Could you check a few things on this model? Use its own coordinates, in mm. Coordinates: 2 decimals unless noted, no trailing zeros. Loops run counter-clockwise (first coordinate to the right, second up) from the corner with the lowest first, then second, coordinate; pieces in that order, holes last. Notation, with made-up numbers: (82.25, 48.25) - (108.25, 48.25) arc R9 cw to (108.25, 62.25) - close; hole circle Ø5 at (54, 69). An arc over 180 degrees is marked (long way). Put each result on its own line as item: value. Start each with the question number.
```python
from build123d import *

# Parameters (mm, degrees)
SKETCH1_W           = 90
SKETCH1_H           = 60
SKETCH1_R           = 4.8
SKETCH1_R_2         = 2.55
BOSS_EXTRUDE1_DEPTH = 6.35
SKETCH3_R           = 1.25
CUT_EXTRUDE1_DEPTH  = 8


with BuildPart() as part:
    # Sketch1 → Boss-Extrude1 (new body)
    with BuildSketch(Plane(origin=(0, 0, 0), x_dir=(1, 0, 0), z_dir=(0, 1, 0))):
        Rectangle(SKETCH1_W, SKETCH1_H)
        with Locations((-37.5, 0)):
            Circle(SKETCH1_R, mode=Mode.SUBTRACT)
        with Locations((37.5, 0)):
            Circle(SKETCH1_R, mode=Mode.SUBTRACT)
        with Locations((-23.6, -23.6)):
            Circle(SKETCH1_R_2, mode=Mode.SUBTRACT)
        with Locations((23.6, -23.6)):
            Circle(SKETCH1_R_2, mode=Mode.SUBTRACT)
        with Locations((23.6, 23.6)):
            Circle(SKETCH1_R_2, mode=Mode.SUBTRACT)
        with Locations((-23.6, 23.6)):
            Circle(SKETCH1_R_2, mode=Mode.SUBTRACT)
    extrude(amount=BOSS_EXTRUDE1_DEPTH)

    # Sketch3 → Cut-Extrude1 (cut)
    with BuildSketch(Plane(origin=(0, 6.35, 0), x_dir=(1, 0, 0), z_dir=(0, 1, 0))):
        with Locations((-11, 0)):
            Circle(SKETCH3_R)
        with Locations((11, 0)):
            Circle(SKETCH3_R)
    extrude(amount=-CUT_EXTRUDE1_DEPTH, mode=Mode.SUBTRACT)


solid = part.part
```
(1) If we mould it in two halves opening along Z, with no side actions, what happens to faces 1 (the flat face through (-1, 3, -30)), 2 (the cylindrical face through (32.705, 3.131, -0.211)), 3 (the cylindrical face through (-21.17, 3.13, -24.37)), 4 (the flat face through (45, 3, 0))? For each: pulls with the +Z half, pulls with the -Z half, needs draft (parallel to the pull), parting line crosses it, or undercut.
(2) I want a section at B-B on z = 0. List the corners of the cut face in (x, y) for me.
(3) I want a section at D-D on y = 2.5. Count the separate pieces of the cut face and the enclosed holes in it, and give its area (3 significant figures).
(4) I want a section at C-C on x = -23.6. List the corners of the cut face in (y, z) for me.
(5) I want a section at A-A on x = 11. List the corners of the cut face in (y, z) for me.
(6) I need wall thicknesses on L1, parallel to X at y = 3.75, z = -23.6; L2, parallel to Z at x = -23.6, y = 1.5; L3, parallel to Z at x = 37.5, y = 4. Which ranges of each line are inside material? Lowest first, please. Write a range as [from, to].
Answer sheet:
1. face 1: pulls with the -Z half
1. face 2: undercut
1. face 3: undercut
1. face 4: needs draft
2. outline: (-45, 0) - (-42.3, 0) - (-42.3, 6.35) - (-45, 6.35) - close; (-32.7, 0) - (-12.25, 0) - (-12.25, 6.35) - (-32.7, 6.35) - close; (-9.75, 0) - (9.75, 0) - (9.75, 6.35) - (-9.75, 6.35) - close; (12.25, 0) - (32.7, 0) - (32.7, 6.35) - (12.25, 6.35) - close; (42.3, 0) - (45, 0) - (45, 6.35) - (42.3, 6.35) - close
3. separate pieces: 1
3. enclosed holes: 8
3. area: 5,160 mm^2
4. outline: (0, -30) - (6.35, -30) - (6.35, -26.15) - (0, -26.15) - close; (0, -21.05) - (6.35, -21.05) - (6.35, 21.05) - (0, 21.05) - close; (0, 26.15) - (6.35, 26.15) - (6.35, 30) - (0, 30) - close
5. outline: (0, -30) - (6.35, -30) - (6.35, -1.25) - (0, -1.25) - close; (0, 1.25) - (6.35, 1.25) - (6.35, 30) - (0, 30) - close
6. L1: x = [-45, -26.15], [-21.05, 21.05], [26.15, 45]
6. L2: z = [-30, -26.15], [-21.05, 21.05], [26.15, 30]
6. L3: z = [-30, -4.8], [4.8, 30]
